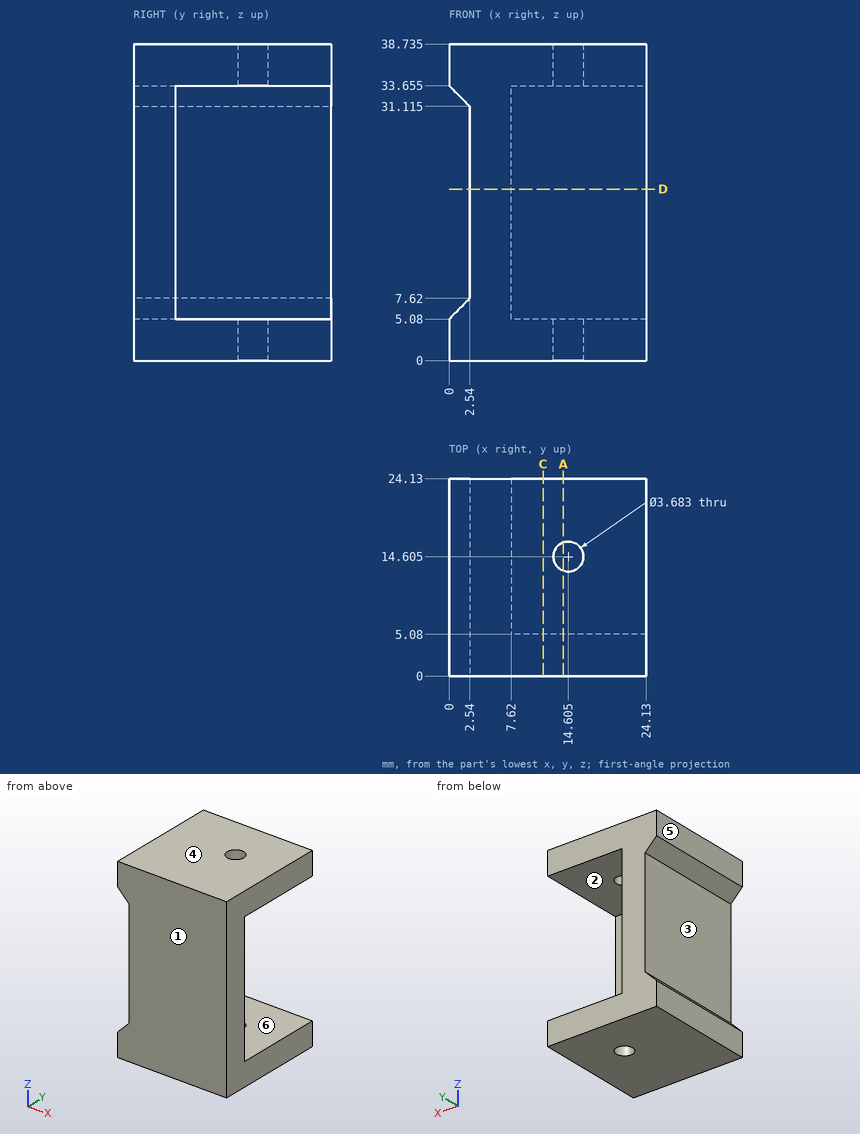
The drawing under review shows one solid part. Ordinate dimensions are in mm from its lowest x, y, z. A direction names the side the tool comes from. Coordinates: 2 decimals unless noted, no trailing zeros. Order: outer loops, then holes, each group sorted by start corner. A loop starts at its lowest first (then second) coordinate and runs counter-clockwise, first axis right, second up. Notation, with made-up numbers: (5, -3.5) -> (30, -3.5) arc R31 ccw to (30, 21.5) -> close; hole circle Ø4 at (88, 30). An arc over 180 degrees is marked (long way). Answer in a Markdown table with one row per item.
(1) Wall thickness on line 1 along Z through (x, y) = (7.75, 22.5) (3 decimals); line 2 along X through (y, z) = (4.5, 10); line 3 along Y through (x, z) = (20.25, 16): over which ranges is each line inside the solid? List them lowest first.
Answers:
| item | result |
|---|---|
| line 1 | 0 to 5.08, 33.655 to 38.735 |
| line 2 | 2.54 to 24.13 |
| line 3 | 0 to 5.08 |
(2) The part is to be moulded in two halves that separate along Z. For the marked faces 4, 5 and 6, say which applies: +Z half, -Z half, draft (parallel to the pull), parting line (faces both ways), or undercut.
Answers:
| item | result |
|---|---|
| face 4 | +Z half |
| face 5 | draft |
| face 6 | undercut |
(3) Machinability: for the marked faces 1, 2 and 3, which of the approach directions +Z, -Z, +X, -X, +Y, -Y give a long, thin tool a straight path to every point of the face, cutting with its end or side? Answer none if there is none.
Answers:
| item | result |
|---|---|
| face 1 | +Z, -Z, +X, -X, -Y |
| face 2 | +X, +Y |
| face 3 | -X, +Y, -Y |
(4) Insertion check: pin 1 (7 mm diameter, centred on y = 7.5, z = 20, fed in from -X); pin 2 (1 mm diameter, centred on y = 8.5, z = 30, fed in from +X); pin 3 (2 mm diameter, centred on x = 14.605, y = 14.605, fed in from +Z). Each pin has a flat end and moves straight along its axis. Give the tip position at first contact, or say it passes through.
Answers:
| item | result |
|---|---|
| pin 1 | x = 2.54 |
| pin 2 | x = 7.62 |
| pin 3 | through |
(5) Consider section C-C (x = 11.5). Write out the cut boundary in (y, z) (3 decimals), plus the area to 3 significant figures.
Answers:
| item | result |
|---|---|
| outline | (0, 0) -> (24.13, 0) -> (24.13, 5.08) -> (5.08, 5.08) -> (5.08, 33.655) -> (24.13, 33.655) -> (24.13, 38.735) -> (0, 38.735) -> close |
| area | 390 mm² |
(6) Consider section D-D (z = 21). Write out the cut boundary in (x, y).
Answers:
| item | result |
|---|---|
| outline | (2.54, 0) -> (24.13, 0) -> (24.13, 5.08) -> (7.62, 5.08) -> (7.62, 24.13) -> (2.54, 24.13) -> close |
(7) Consider section A-A (x = 14). Write out the cut boundary in (y, z) (3 decimals).
Answers:
| item | result |
|---|---|
| outline | (0, 0) -> (12.866, 0) -> (12.866, 5.08) -> (5.08, 5.08) -> (5.08, 33.655) -> (12.866, 33.655) -> (12.866, 38.735) -> (0, 38.735) -> close; (16.344, 0) -> (24.13, 0) -> (24.13, 5.08) -> (16.344, 5.08) -> close; (16.344, 33.655) -> (24.13, 33.655) -> (24.13, 38.735) -> (16.344, 38.735) -> close |
